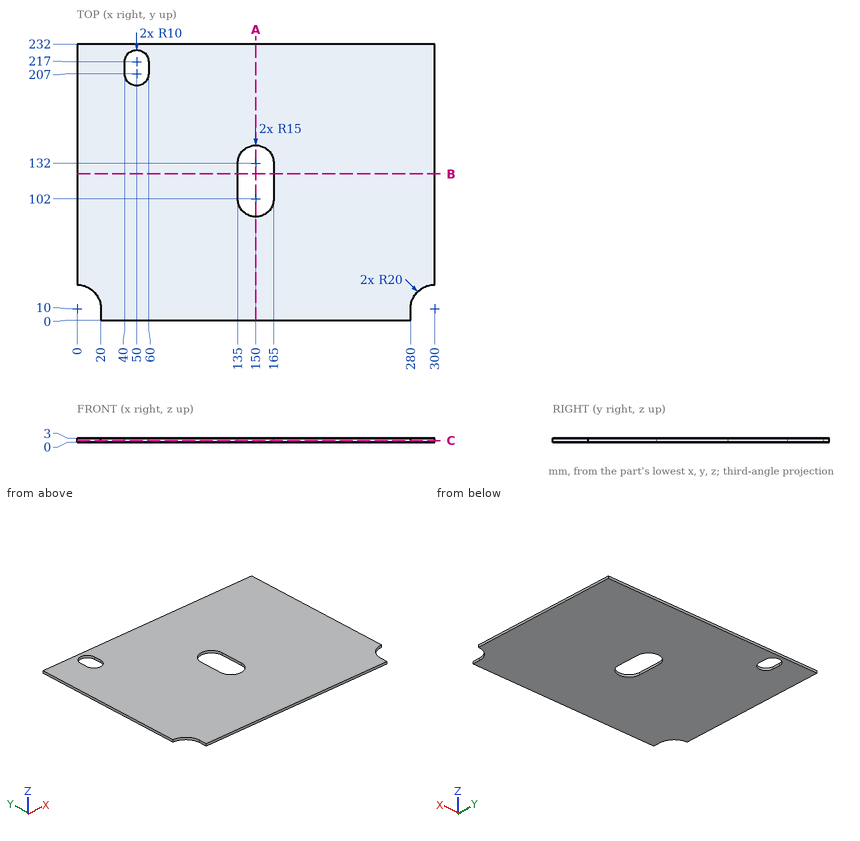
Study the drawing (mm; zero at the part's minimum x, y, z) and answer. Round coordinates to 2 decimals unless told otherwise and drop trailing zeros. Write each loop counter-clockwise with the first axis right and the second up, starting at its lowest first coordinate (ties: lowest second). Pieces come first, ordered by that corner, then holes. Notation, with made-up numbers: (83.5, 50) -> (120.5, 50) arc R21 cw to (120.5, 67) -> close; hole circle Ø10 at (58, 40.5). An arc over 180 degrees is marked (long way). Use CSV: the item, a comma, the result in double quotes. Start each with the question number.
(1) Section C-C on z = 1.25 is taken. Give the vertices of the cut face in (x, y).
(2) Section B-B on y = 123 is taken. Give the vertices of the cut face in (x, z), then the cut area to 3 significant figures.
(3) Consider L1, parallel to X at y = 217, z = 1.2; L2, parallel to X at y = 114.5, z = 2.75; L3, parallel to Y at x = 153, z = 0.5. Determine where each line is inside the solid, lowest interval first. Write a range as from..to.
(4) Section A-A on x = 150 is taken. Give the vertices of the cut face in (y, z), then the cut area to 3 significant figures.
A:
1,outline,"(0, 30) arc R20 cw to (20, 10) -> (20, 0) -> (280, 0) -> (280, 10) arc R20 cw to (300, 30) -> (300, 232) -> (0, 232) -> close; hole (40, 207) arc R10 ccw to (60, 207) -> (60, 217) arc R10 ccw to (40, 217) -> close; hole (135, 102) arc R15 ccw to (165, 102) -> (165, 132) arc R15 ccw to (135, 132) -> close"
2,outline,"(0, 0) -> (135, 0) -> (135, 3) -> (0, 3) -> close; (165, 0) -> (300, 0) -> (300, 3) -> (165, 3) -> close"
2,area,"810 mm²"
3,L1,"x = 0..40, 60..300"
3,L2,"x = 0..135, 165..300"
3,L3,"y = 0..87.3, 146.7..232"
4,outline,"(0, 0) -> (87, 0) -> (87, 3) -> (0, 3) -> close; (147, 0) -> (232, 0) -> (232, 3) -> (147, 3) -> close"
4,area,"516 mm²"
